Could you check a few things on this model? Use its own coordinates, in mm. A direction names the side the tool comes from. Coordinates: 2 decimals unless noted, no trailing zeros. Order: outer loops, then holes, each group sorted by start corner. A loop starts at its lowest first (then second) coordinate and runs counter-clockwise, first axis right, second up. Notation, with made-up numbers: M 32,10 L 38,10 A19 ccw 38,27 Z; hole C -11.75,26 d4. An arc over 180 degrees is marked long. Write item = value, one per line. Start each with the question number.
from build123d import *

# Parameters (mm, degrees)
SKETCH001_W     = 298
SKETCH001_H     = 108
PAD_DEPTH       = 9.5
SKETCH002_W     = 287
SKETCH002_H     = 97
POCKET_DEPTH    = 8
SKETCH003_W     = 299
SKETCH003_H     = 109
SKETCH003_W_2   = 294.96
SKETCH003_H_2   = 104.96
POCKET001_DEPTH = 1.7
SKETCH004_W     = 80
SKETCH004_H     = 4
SKETCH004_W_2   = 4
SKETCH004_H_2   = 32.5
POCKET002_DEPTH = 1
SKETCH005_W     = 12
SKETCH005_H     = 3.5
POCKET003_DEPTH = 15
SKETCH_W        = 12
SKETCH_H        = 6
POCKET004_DEPTH = 5.5
FILLET_R        = 1.5
FILLET001_R     = 1
FILLET002_R     = 1
FILLET003_R     = 1
FILLET004_R     = 1
FILLET005_R     = 1


with BuildPart() as part:
    # Sketch001 → Pad (new body)
    with BuildSketch(Plane.XY):
        Rectangle(SKETCH001_W, SKETCH001_H)
    extrude(amount=PAD_DEPTH)

    # Sketch002 (on Face6 of Pad) → Pocket (cut)
    with BuildSketch(Plane.XY.offset(9.5)):
        Rectangle(SKETCH002_W, SKETCH002_H)
    extrude(amount=-POCKET_DEPTH, mode=Mode.SUBTRACT)

    # Sketch003 (on Face5 of Pocket) → Pocket001 (cut)
    with BuildSketch(Plane.XY.offset(9.5)):
        Rectangle(SKETCH003_W, SKETCH003_H)
        Rectangle(SKETCH003_W_2, SKETCH003_H_2, mode=Mode.SUBTRACT)
    extrude(amount=-POCKET001_DEPTH, mode=Mode.SUBTRACT)

    # Sketch004 (on Face11 of Pocket001) → Pocket002 (cut)
    with BuildSketch(Plane.XY.offset(9.5)):
        with Locations((-95, 50.5)):
            Rectangle(SKETCH004_W, SKETCH004_H)
        with Locations((0, 50.5)):
            Rectangle(SKETCH004_W, SKETCH004_H)
        with Locations((95, 50.5)):
            Rectangle(SKETCH004_W, SKETCH004_H)
        with Locations((95, -50.5)):
            Rectangle(SKETCH004_W, SKETCH004_H)
        with Locations((0, -50.5)):
            Rectangle(SKETCH004_W, SKETCH004_H)
        with Locations((-95, -50.5)):
            Rectangle(SKETCH004_W, SKETCH004_H)
        with Locations((-145.5, 23.75)):
            Rectangle(SKETCH004_W_2, SKETCH004_H_2)
        with Locations((-145.5, -23.75)):
            Rectangle(SKETCH004_W_2, SKETCH004_H_2)
        with Locations((145.5, 23.75)):
            Rectangle(SKETCH004_W_2, SKETCH004_H_2)
        with Locations((145.5, -23.75)):
            Rectangle(SKETCH004_W_2, SKETCH004_H_2)
    extrude(amount=-POCKET002_DEPTH, mode=Mode.SUBTRACT)

    # Sketch005 (on Face1 of Pocket002) → Pocket003 (cut)
    with BuildSketch(Plane(origin=(0, 54, 0), x_dir=(-1, 0, 0), z_dir=(0, 1, 0))):
        with Locations((124.3, 2.5)):
            Rectangle(SKETCH005_W, SKETCH005_H)
    extrude(amount=-POCKET003_DEPTH, mode=Mode.SUBTRACT)

    # Sketch (on Face1 of Pocket003) → Pocket004 (cut)
    with BuildSketch(Plane(origin=(0, 54, 0), x_dir=(-1, 0, 0), z_dir=(0, 1, 0))):
        with Locations((124.3, 3)):
            Rectangle(SKETCH_W, SKETCH_H)
    extrude(amount=-POCKET004_DEPTH, mode=Mode.SUBTRACT)

    # Fillet
    fillet_edges = [part.edges().sort_by_distance(p)[0] for p in [
        (-149, 54, 3.9),
        (-149, -54, 3.9),
        (149, 54, 3.9),
        (149, -54, 3.9),
    ]]
    fillet(fillet_edges, radius=FILLET_R)

    # Fillet001
    fillet001_edges = [part.edges().sort_by_distance(p)[0] for p in [
        (147.48, -52.48, 8.65),
        (-147.48, -52.48, 8.65),
        (147.48, 52.48, 8.65),
        (-147.48, 52.48, 8.65),
    ]]
    fillet(fillet001_edges, radius=FILLET001_R)

    # Fillet002
    fillet002_edges = [part.edges().sort_by_distance(p)[0] for p in [
        (143.5, 48.5, 5.5),
        (-143.5, 48.5, 5.5),
        (-143.5, -48.5, 5.5),
        (143.5, -48.5, 5.5),
    ]]
    fillet(fillet002_edges, radius=FILLET002_R)

    # Fillet003
    fillet003_edges = [part.edges().sort_by_distance(p)[0] for p in [
        (143.5, 40, 9),
        (135, 48.5, 9),
        (55, 48.5, 9),
        (40, 48.5, 9),
        (143.5, -7.5, 9),
        (143.5, 7.5, 9),
        (143.5, -40, 9),
        (135, -48.5, 9),
        (40, -48.5, 9),
        (-55, -48.5, 9),
        (-40, 48.5, 9),
        (-55, 48.5, 9),
        (-135, 48.5, 9),
        (-143.5, 40, 9),
        (-143.5, -7.5, 9),
        (-143.5, 7.5, 9),
        (-143.5, -40, 9),
        (-135, -48.5, 9),
        (-40, -48.5, 9),
        (55, -48.5, 9),
    ]]
    fillet(fillet003_edges, radius=FILLET003_R)

    # Fillet004
    fillet004_edges = [part.edges().sort_by_distance(p)[0] for p in [
        (-118.3, 51.25, 6),
        (-130.3, 51.25, 6),
    ]]
    fillet(fillet004_edges, radius=FILLET004_R)

    # Fillet005
    fillet005_edges = [part.edges().sort_by_distance(p)[0] for p in [
        (0, -54, 0),
    ]]
    fillet(fillet005_edges, radius=FILLET005_R)


solid = part.part
(1) Please list where these lines run through material, in increasing order: probe 1 along Y at (x, z) = (79, 7); probe 2 along Y at (x, z) = (4.5, 8.25); probe 3 along X at (y, z) = (36, 6.75). Write a range as from..to.
(2) Thinking about a two-plate mould opening in Y: for faces 1 (the flat face through (-2, 1, 1.5)), 2 (the flat face through (143, 49, 9.5)), 3 (the flat face through (-2, 54, 4)), 4 (the flat face through (-2, -54, 4)), which applies, released by +Y, released by -Y, zero draft, split by the parting line, or undercut?
(3) Will these pins go through, and if not, where does the flat tip stop? P1, Ø2, axis at x = 67, y = 38, coming from the +Z side; P2, Ø0.8, axis at x = 146, z = 9, coming from the +Y side; P3, Ø1.5, axis at y = 22.5, z = 8, coming from the -X side; P4, Ø7.5, axis at x = -122, y = 45.5, coming from the +Z side.
(4) Imagine slicing it at B-B on y = -19. List the corners of the cut face in (x, z) for me.
(5) For faces 5 (the flat face through (-2, -48.5, 5)), 6 (the flat face through (-130.3, 50, 2)), 7 (the flat face through (-124, 51, 6)), 8 (the flat face through (-124, 44, 0.75)), which set-ups out of +Z, -Z, +X, -X, +Y, -Y let a thin tool reach every point of the face, with its end or its side?
(6) Imagine slicing it at C-C on x = -48. List the corners of the cut face in (y, z) for me, plus the area to 3 significant figures.
(7) Imagine slicing it at A-A on x = -122. List the corners of the cut face in (y, z) for me, plus the area to 3 significant figures.
Response:
q1.probe_1 = -54..-48.5, 48.5..54
q1.probe_2 = -52.48..-48.5, 48.5..52.48
q1.probe_3 = -149..-143.5, 143.5..149
q2.face_1 = undercut
q2.face_2 = zero draft
q2.face_3 = released by +Y
q2.face_4 = released by -Y
q3.P1 = 1.5
q3.P2 = 52.48
q3.P3 = -149
q3.P4 = 8.5
q4.outline = M -149,1 A1 ccw -148,0 L 148,0 A1 ccw 149,1 L 149,7.8 L 147.48,7.8 L 147.48,8.5 L 143.5,8.5 L 143.5,1.5 L -143.5,1.5 L -143.5,8.5 L -147.48,8.5 L -147.48,7.8 L -149,7.8 Z
q5.face_5 = +Z
q5.face_6 = +Y
q5.face_7 = -Z, +Y
q5.face_8 = +Z, +Y
q6.outline = M -54,1 A1 ccw -53,0 L 53,0 A1 ccw 54,1 L 54,7.8 L 52.48,7.8 L 52.48,9.5 L 48.5,9.5 L 48.5,1.5 L -48.5,1.5 L -48.5,9.5 L -52.48,9.5 L -52.48,7.8 L -54,7.8 Z
q6.area = 244 mm2
q7.outline = M -54,1 A1 ccw -53,0 L 48.5,0 L 48.5,0.75 L 39,0.75 L 39,1.5 L -48.5,1.5 L -48.5,8.5 L -52.48,8.5 L -52.48,7.8 L -54,7.8 Z; M 48.5,6 L 54,6 L 54,7.8 L 52.48,7.8 L 52.48,8.5 L 48.5,8.5 Z
q7.area = 197 mm2
